The model under review builds one solid part; all positions refer to its coordinate system, in mm. Face numbers are marked on the shaded views. A direction names the side the tool comes from. Round coordinates to 2 decimals unless told otherwise and drop trailing zeros. Write each loop counter-clockwise with the first axis right and the second up, starting at its lowest first coordinate (ties: lowest second). Pieces come first, ordered by that corner, then holes. Notation, with made-up numbers: M -10.5,46 L 31.5,46 A27 cw 31.5,80 Z; hole C 74,27.25 d1. An arc over 180 degrees is marked long. Write item = value, one per line. Start each with the question number.
Item 1: To check wall thickness, follow line 1 along Y through (x, z) = (-9, 19.75); line 2 along Z through (x, y) = (-22, -12). State the ranges of each line that lie inside material, in increasing order.
Item 2: Tool access review of the marked faces 4 and 5: name each direction out of +Z, -Z, +X, -X, +Y, -Y from which nothing blocks a thin tool from reaching the whole face with its end or side.
Item 3: Take a section at C-C, the plane y = -17.5. Give the boundary of the cut face in (x, z).
Item 4: The part is to be moulded in two halves that separate along Z. For the marked faces 1, 2 and 3, say which applies: +Z half, -Z half, draft (parallel to the pull), parting line (faces both ways), or undercut.
Item 5: Take a section at B-B, the plane x = 12. Give the boundary of the cut face in (y, z), plus the area to 3 significant figures.
Item 6: Take a section at A-A, the plane z = 19.25. Give the boundary of the cut face in (x, y), plus the area to 3 significant figures.
Item 7: For pin 1 Ø8 at (x, y) = (6, 15.5) entering from +Z, flat-tipped, find the tip position at first contact; note if it passes through.
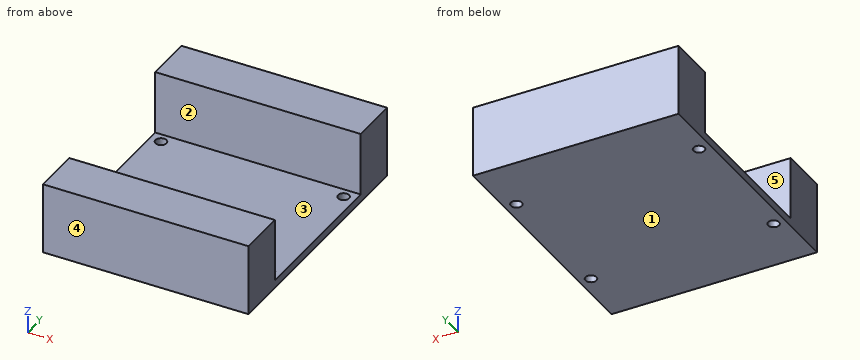
from build123d import *

# Parameters (mm, degrees)
F0_W     = 66.04
F0_H     = 81.077
F1_DEPTH = 2.54
F2_W     = 66.04
F2_H     = 15.383
F3_DEPTH = 20.371
F4_R     = 1.778
F5_DEPTH = 25


with BuildPart() as f1:
    # F0 (on Top) → F1 (new body)
    with BuildSketch(Plane.XY):
        Rectangle(F0_W, F0_H)
    extrude(amount=F1_DEPTH)

    # F2 (on face) → F3 (join)
    with BuildSketch(Plane.XY.offset(2.54)):
        with Locations((0, 32.847)):
            Rectangle(F2_W, F2_H)
        with Locations((0, -32.847)):
            Rectangle(F2_W, F2_H)
    extrude(amount=F3_DEPTH)

    # F4 (on face) → F5 (cut)
    with BuildSketch(Plane.XY.offset(2.54)):
        with Locations((-29.337, 21.8285)):
            Circle(F4_R)
        with Locations((29.337, 21.8285)):
            Circle(F4_R)
        with Locations((29.337, -21.8285)):
            Circle(F4_R)
        with Locations((-29.337, -21.8285)):
            Circle(F4_R)
    extrude(amount=-F5_DEPTH, mode=Mode.SUBTRACT)


solid = f1.part
Response values:
q1.line_1 = -40.54 to -25.16, 25.16 to 40.54
q1.line_2 = 0 to 2.54
q2.face_4 = +Z, -Z, +X, -X, -Y
q2.face_5 = +Z, +X, -X
q3.outline = M -33.02,0 L 33.02,0 L 33.02,2.54 L -33.02,2.54 Z
q4.face_1 = -Z half
q4.face_2 = draft
q4.face_3 = +Z half
q5.outline = M -40.54,0 L 40.54,0 L 40.54,22.91 L 25.16,22.91 L 25.16,2.54 L -25.16,2.54 L -25.16,22.91 L -40.54,22.91 Z
q5.area = 833 mm2
q6.outline = M -33.02,-40.54 L 33.02,-40.54 L 33.02,-25.16 L -33.02,-25.16 Z; M -33.02,25.16 L 33.02,25.16 L 33.02,40.54 L -33.02,40.54 Z
q6.area = 2,030 mm2
q7.pin_1 = 2.54
